from build123d import *

# Parameters (mm, degrees)
SKETCH1_R           = 32
BOSS_EXTRUDE1_DEPTH = 15
SKETCH2_R           = 22.5
CUT_EXTRUDE1_DEPTH  = 3
SKETCH3_R           = 7.5
BOSS_EXTRUDE2_DEPTH = 2
SKETCH4_R           = 24.5
CUT_EXTRUDE2_DEPTH  = 11
SKETCH5_R           = 5
BOSS_EXTRUDE3_DEPTH = 15
SKETCH6_RX          = 5
SKETCH6_RY          = 4
CUT_EXTRUDE3_DEPTH  = 48.675989764
SKETCH7_R           = 3
CUT_EXTRUDE4_DEPTH  = 1
CUT_EXTRUDE5_DEPTH  = 7


with BuildPart() as part:
    # Sketch1 → Boss-Extrude1 (new body)
    with BuildSketch(Plane(origin=(0, 0, 0), x_dir=(1, 0, 0), z_dir=(0, 1, 0))):
        with Locations(Location((0, 0, 0), (0, 0, 270))):
            Circle(SKETCH1_R)
    extrude(amount=BOSS_EXTRUDE1_DEPTH)

    # Sketch2 → Cut-Extrude1 (cut)
    with BuildSketch(Plane.XZ):
        with Locations(Location((0, 0, 0), (0, 0, 270))):
            Circle(SKETCH2_R)
    extrude(amount=-CUT_EXTRUDE1_DEPTH, mode=Mode.SUBTRACT)

    # Sketch3 → Boss-Extrude2 (add)
    with BuildSketch(Plane.XZ.offset(-3)):
        with Locations(Location((0, 0, 0), (0, 0, 270))):
            Circle(SKETCH3_R)
    extrude(amount=BOSS_EXTRUDE2_DEPTH)

    # Sketch4 → Cut-Extrude2 (cut)
    with BuildSketch(Plane(origin=(0, 15, 0), x_dir=(1, 0, 0), z_dir=(0, 1, 0))):
        with Locations(Location((0, 0, 0), (0, 0, 270))):
            Circle(SKETCH4_R)
    extrude(amount=-CUT_EXTRUDE2_DEPTH, mode=Mode.SUBTRACT)

    # Sketch5 → Boss-Extrude3 (add)
    with BuildSketch(Plane(origin=(0, 4, 0), x_dir=(1, 0, 0), z_dir=(0, 1, 0))):
        with Locations(Location((0, 0, 0), (0, 0, 270))):
            Circle(SKETCH5_R)
    extrude(amount=BOSS_EXTRUDE3_DEPTH)

    # Sketch6 → Cut-Extrude3 (cut, through all)
    with BuildSketch(Plane(origin=(0, 4, 0), x_dir=(1, 0, 0), z_dir=(0, 1, 0))):
        with Locations(Location((0, -14.5), (0, 0, -90))):
            Ellipse(SKETCH6_RX, SKETCH6_RY)
        with Locations(Location((-10.253048327, -10.253048327), (0, 0, -135))):
            Ellipse(SKETCH6_RX, SKETCH6_RY)
        with Locations(Location((-14.5, 0), (0, 0, 180))):
            Ellipse(SKETCH6_RX, SKETCH6_RY)
        with Locations(Location((-10.253048327, 10.253048327), (0, 0, 135))):
            Ellipse(SKETCH6_RX, SKETCH6_RY)
        with Locations(Location((0, 14.5), (0, 0, 90))):
            Ellipse(SKETCH6_RX, SKETCH6_RY)
        with Locations(Location((10.253048327, 10.253048327), (0, 0, -135))):
            Ellipse(SKETCH6_RX, SKETCH6_RY)
        with Locations(Location((14.5, 0), (0, 0, 0))):
            Ellipse(SKETCH6_RX, SKETCH6_RY)
        with Locations(Location((10.253048327, -10.253048327), (0, 0, -45))):
            Ellipse(SKETCH6_RX, SKETCH6_RY)
    extrude(amount=-CUT_EXTRUDE3_DEPTH, mode=Mode.SUBTRACT)

    # Sketch7 → Cut-Extrude4 (cut)
    with BuildSketch(Plane(origin=(0, 19, 0), x_dir=(1, 0, 0), z_dir=(0, 1, 0))):
        with Locations(Location((0, 0, 0), (0, 0, 270))):
            Circle(SKETCH7_R)
    extrude(amount=-CUT_EXTRUDE4_DEPTH, mode=Mode.SUBTRACT)

    # Sketch8 → Cut-Extrude5 (cut)
    with BuildSketch(Plane(origin=(0, 18, 0), x_dir=(1, 0, 0), z_dir=(0, 1, 0))):
        with BuildLine():
            Line((2, -1.5), (2, 1.5))
            ThreePointArc((2, 1.5), (0, 2.5), (-2, 1.5))
            Line((-2, 1.5), (-2, -1.5))
            ThreePointArc((-2, -1.5), (0, -2.5), (2, -1.5))
        make_face()
    extrude(amount=-CUT_EXTRUDE5_DEPTH, mode=Mode.SUBTRACT)


solid = part.part
Here's how the part is built. I have some questions about the finished solid (model axes, mm). A direction names the side the tool comes from. Give positions to 0.01 mm unless a question says otherwise; leave off trailing zeros. Order: outer loops, then holes, each group sorted by start corner. A loop starts at its lowest first (then second) coordinate and runs counter-clockwise, first axis right, second up. Notation, with made-up numbers: (-12.75, 41) -> (35.25, 41) arc R26 cw to (35.25, 64) -> close; hole circle Ø1 at (-31.5, 88). An arc over 180 degrees is marked (long way). Use a Markdown table: item, result. Add a question column.
Item 1: Will these pins go through, and if not, where does the flat tip stop? pin 1 (5 mm diameter, centred on x = -19, y = 12.5, fed in from -Z); pin 2 (3.5 mm diameter, centred on x = 0, z = 0, fed in from +Y); pin 3 (14.5 mm diameter, centred on x = 11, z = -10.5, fed in from +Y).
Item 2: I need wall thicknesses on line 1 (X direction, y = 1.4, z = 0); line 2 (X direction, y = 10.25, z = 0); line 3 (X direction, y = 18.75, z = 0). Which ranges of each line are inside material? Lowest first, please.
Item 3: Imagine slicing it at A-A on y = 7. Please give me the cut outline in (x, z).
Item 4: If we mould it in two halves opening along X, with no side actions, what happens to faces 4 (the face through (-31.24, 7.4, -6.94)), 5 (the face through (-4.88, 11.4, -1.08)), 6 (the face through (-3.3, 19, -0.1)), 7 (the face through (6, 4, 0))? For each: pulls with the +X half, pulls with the -X half, needs draft (parallel to the pull), parting line crosses it, or undercut.
Item 5: For faces 1 (the face through (0, 11, 0)), 2 (the face through (-7, 0, -22)), 3 (the face through (0, 1, 0)), which set-ups out of +Z, -Z, +X, -X, +Y, -Y let a thin tool reach every point of the face, with its end or its side?
Item 6: Imagine slicing it at B-B on z = 0. Give the number of separate pieces and of enclosed holes in the cut face, plus the area to 3 significant figures.
Data:
| question | item | result |
|---|---|---|
| 1 | pin 1 | stops at z = -27.42 |
| 1 | pin 2 | stops at y = 11 |
| 1 | pin 3 | stops at y = 4 |
| 2 | line 1 | x = -32 to -22.5, -7.5 to 7.5, 22.5 to 32 |
| 2 | line 2 | x = -32 to -24.5, -5 to 5, 24.5 to 32 |
| 2 | line 3 | x = -5 to -3, 3 to 5 |
| 3 | outline | circle Ø64 at (0, 0); circle Ø10 at (0, 0); hole circle Ø49 at (0, 0) |
| 4 | face 4 | parting line crosses it |
| 4 | face 5 | undercut |
| 4 | face 6 | needs draft |
| 4 | face 7 | undercut |
| 5 | face 1 | +Y |
| 5 | face 2 | +Z, -Z, +X, -X, -Y |
| 5 | face 3 | -Y |
| 6 | separate pieces | 3 |
| 6 | enclosed holes | 0 |
| 6 | area | 412 mm² |
